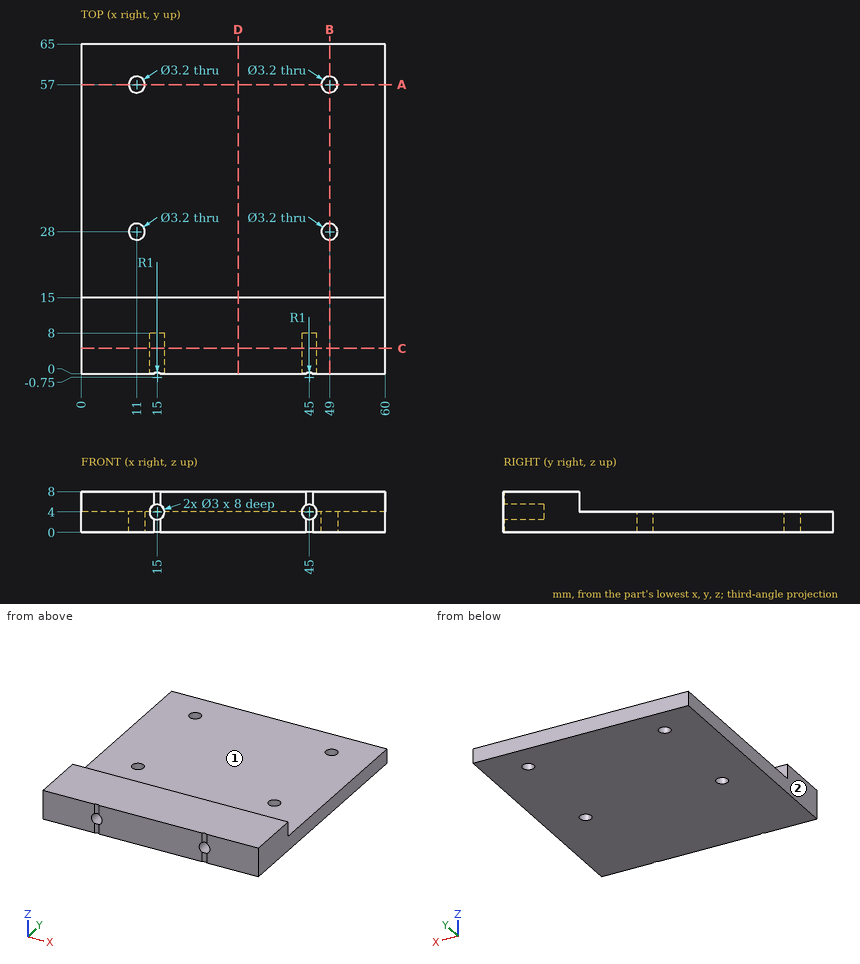
Job drawing, mm, ordinate dimensions from the low corner. One solid piece. A direction names the side the tool comes from. Give positions to 0.01 mm unless a question says otherwise; leave off trailing zeros. Loops run counter-clockwise (first coordinate to the right, second up) from the corner with the lowest first, then second, coordinate; pieces in that order, holes last. Notation, with made-up numbers: (1.5, 36) -> (60.5, 36) arc R21 cw to (60.5, 57) -> close; hole circle Ø8 at (37.5, 60.25). An arc over 180 degrees is marked (long way). Write each question's results on one line, items separated by ' | '. Start each with the question number.
Q1. Band-saw the part on B-B on x = 49. List the corners of the cut face in (y, z), plus the area to 3 significant figures.
Q2. Wall check: L1, parallel to Y at x = 49, z = 1.65; L2, parallel to Z at x = 45, y = 3; L3, parallel to Y at x = 48, z = 6.5. Give the ranges that are in metal, low to high.
Q3. Band-saw the part on A-A on y = 57. List the corners of the cut face in (x, z), plus the area to 3 significant figures.
Q4. Which spindle directions (+Z, -Z, +X, -X, +Y, -Y) get a long thin tool onto all of the face, cutting with end or side? Do the marked faces 1 and 2. Say none if no direction does.
Q5. Band-saw the part on D-D on x = 31. List the corners of the cut face in (y, z), plus the area to 3 significant figures.
Q6. Band-saw the part on C-C on y = 5. List the corners of the cut face in (x, z).
Q7. Pin check, flat tips, straight feed: P1, Ø2.5, axis at x = 49, y = 28, coming from the +Z side; P2, Ø5, axis at x = 49, y = 57, coming from the +Z side; P3, Ø0.9, axis at x = 14.5, z = 4.5, coming from the -Y side. Stop position of each tip, or through.
Results are:
1) outline: (0, 0) -> (26.4, 0) -> (26.4, 4) -> (15, 4) -> (15, 8) -> (0, 8) -> close; (29.6, 0) -> (55.4, 0) -> (55.4, 4) -> (29.6, 4) -> close; (58.6, 0) -> (65, 0) -> (65, 4) -> (58.6, 4) -> close | area: 294 mm²
2) L1: y = 0 to 26.4, 29.6 to 55.4, 58.6 to 65 | L2: z = 0 to 2.5, 5.5 to 8 | L3: y = 0 to 15
3) outline: (0, 0) -> (9.4, 0) -> (9.4, 4) -> (0, 4) -> close; (12.6, 0) -> (47.4, 0) -> (47.4, 4) -> (12.6, 4) -> close; (50.6, 0) -> (60, 0) -> (60, 4) -> (50.6, 4) -> close | area: 214 mm²
4) face 1: +Z, +X, -X, +Y | face 2: +Z, -Z, -X, +Y, -Y
5) outline: (0, 0) -> (65, 0) -> (65, 4) -> (15, 4) -> (15, 8) -> (0, 8) -> close | area: 320 mm²
6) outline: (0, 0) -> (60, 0) -> (60, 8) -> (0, 8) -> close; hole circle Ø3 at (15, 4); hole circle Ø3 at (45, 4)
7) P1: passes through | P2: stops at z = 4 | P3: stops at y = 8
